```python
from build123d import *

# Parameters (mm, degrees)
F1_DEPTH = 3


with BuildPart() as f1:
    # F0 (on Front) → F1 (new body)
    with BuildSketch(Plane.XZ):
        with BuildLine():
            Line((-45.218005, 34.439229), (-45.218005, 49.439229))
            ThreePointArc((-45.218005, 49.439229), (-63.703917, 28.74503), (-43.718005, 9.495558))
            Line((-43.718005, 9.495558), (-3.718005, 9.495558))
            Line((-3.718005, 9.495558), (7.654663, 1.584798))
            ThreePointArc((7.654663, 1.584798), (8.427256, -0.635059), (6.55539, -2.0566))
            Line((6.55539, -2.0566), (-9.47062, -2.399568))
            ThreePointArc((-9.47062, -2.399568), (-15.016504, -4.801726), (-17.299454, -10.397736))
            Line((-17.299454, -10.397736), (-17.299454, -13.56711))
            Line((-17.299454, -13.56711), (18.700546, -13.56711))
            ThreePointArc((18.700546, -13.56711), (21.528974, -12.395537), (22.700546, -9.56711))
            Line((22.700546, -9.56711), (22.700546, -1.56711))
            Line((22.700546, -1.56711), (7.843316, 24.495558))
            ThreePointArc((7.843316, 24.495558), (2.843316, 27.400627), (-2.156684, 24.495558))
            Line((-2.156684, 24.495558), (-30.731795, 44.706027))
            ThreePointArc((-30.731795, 44.706027), (-36.098072, 47.987087), (-42.218005, 49.439229))
            Line((-42.218005, 49.439229), (-42.218005, 34.439229))
            Line((-42.218005, 34.439229), (-45.218005, 34.439229))
        make_face()
    extrude(amount=-F1_DEPTH)


solid = f1.part
```
Can you work these out from the model? Positions are in its coordinate system, mm. A direction names the side the tool comes from. Coordinates: 2 decimals unless noted, no trailing zeros. Loops run counter-clockwise (first coordinate to the right, second up) from the corner with the lowest first, then second, coordinate; pieces in that order, holes last. Notation, with made-up numbers: (42.5, -9.75) -> (80.5, -9.75) arc R23 cw to (80.5, 6.25) -> close; hole circle Ø1 at (77, 26.5). An arc over 180 degrees is marked (long way). Put each result on its own line as item: value. Start each with the question number.
Q1. Thinking about a two-plate mould opening in X: for faces 4 (the face through (-45.218, 1, 42)), 5 (the face through (-24, 1, 9.496)), 6 (the face through (22.701, 1, -6)), which applies, pulls with the +X half, pulls with the -X half, needs draft (parallel to the pull), parting line crosses it, or undercut?
Q2. I'm going to push flat-ended pins straight in: P1, Ø0.9, axis at y = 2, z = -12, coming from the -X side; P2, Ø1.5, axis at x = -30.5, y = 2.5, coming from the -Z side; P3, Ø1.5, axis at y = 2, z = 41.5, coming from the -X side. Where does each tip first touch, or does it pass through?
Q3. For faces 1 (the face through (-17.299, 1, -12)), 2 (the face through (-14.955, 1.479, -4.74)), 3 (the face through (-44, 1, 34.439)), which set-ups out of +Z, -Z, +X, -X, +Y, -Y let a thin tool reach every point of the face, with its end or its side?
Q4. I want a section at B-B (y = 1.85). Write out the boundary of the cut face in (x, z), plus the area to 3 significant figures.
Q5. I want a section at D-D (x = -57.5). Write out the boundary of the cut face in (y, z).
Q6. I want a section at C-C (z = 13.5). Write out the boundary of the cut face in (x, y).
Q7. I want a section at A-A (x = 2). Write out the boundary of the cut face in (y, z).
Q8. If I drill on line 1 (Z direction, x = -14, y = 0.65); line 2 (Z direction, x = 4, y = 1.9); line 3 (X direction, y = 1.4, z = 44), over which ranges is the centre line in solid material (lowest first)? Write a range as [from, to].
Taken from the geometry:
1. face 4: undercut
1. face 5: needs draft
1. face 6: pulls with the +X half
2. P1: stops at x = -17.3
2. P2: stops at z = 9.5
2. P3: stops at x = -60.25
3. face 1: -Z, -X, +Y, -Y
3. face 2: -X, +Y, -Y
3. face 3: +Z, +Y, -Y
4. outline: (-45.22, 34.44) -> (-45.22, 49.44) arc R20 ccw to (-43.72, 9.5) -> (-3.72, 9.5) -> (7.65, 1.58) arc R2 cw to (6.56, -2.06) -> (-9.47, -2.4) arc R8 ccw to (-17.3, -10.4) -> (-17.3, -13.57) -> (18.7, -13.57) arc R4 ccw to (22.7, -9.57) -> (22.7, -1.57) -> (7.84, 24.5) arc R5.76 ccw to (-2.16, 24.5) -> (-30.73, 44.71) arc R20 ccw to (-42.22, 49.44) -> (-42.22, 34.44) -> close
4. area: 2,660 mm2
5. outline: (0, 15) -> (3, 15) -> (3, 43.99) -> (0, 43.99) -> close
6. outline: (-55.72, 0) -> (14.11, 0) -> (14.11, 3) -> (-55.72, 3) -> close
7. outline: (0, -13.57) -> (3, -13.57) -> (3, -2.15) -> (0, -2.15) -> close; (0, 5.52) -> (3, 5.52) -> (3, 27.34) -> (0, 27.34) -> close
8. line 1: z = [-13.57, -3.92], [9.5, 32.87]
8. line 2: z = [-13.57, -2.11], [4.13, 27.28]
8. line 3: x = [-57.49, -45.22], [-42.22, -29.73]
